from build123d import *

# Parameters (mm, degrees)
F0_W     = 127
F0_H     = 88.9
F1_DEPTH = 127
F2_R     = 5.08
F4_DEPTH = 114.3
F6_DEPTH = 10.16


with BuildPart() as f1:
    # F0 (on Top) → F1 (new body)
    with BuildSketch(Plane.XY):
        with Locations((4.240815, 7.625027)):
            Rectangle(F0_W, F0_H)
    extrude(amount=F1_DEPTH)

    # F2
    f2_edges = [f1.edges().sort_by_distance(p)[0] for p in [
        (-59.259185, -36.824973, 63.5),
        (67.740815, -36.824973, 63.5),
        (67.740815, 52.075027, 63.5),
        (-59.259185, 52.075027, 63.5),
    ]]
    fillet(f2_edges, radius=F2_R)

    # F3 (on face) → F4 (cut)
    with BuildSketch(Plane.XY.offset(127)):
        with BuildLine():
            Line((58.850815, 49.535027), (-50.369185, 49.535027))
            ThreePointArc((-50.369185, 49.535027), (-54.859313, 47.675155), (-56.719185, 43.185027))
            Line((-56.719185, 43.185027), (-56.719185, -27.934973))
            ThreePointArc((-56.719185, -27.934973), (-54.859313, -32.425101), (-50.369185, -34.284973))
            Line((-50.369185, -34.284973), (58.850815, -34.284973))
            ThreePointArc((58.850815, -34.284973), (63.340943, -32.425101), (65.200815, -27.934973))
            Line((65.200815, -27.934973), (65.200815, 43.185027))
            ThreePointArc((65.200815, 43.185027), (63.340943, 47.675155), (58.850815, 49.535027))
        make_face()
    extrude(amount=-F4_DEPTH, mode=Mode.SUBTRACT)

    # F5 (on face) → F6 (cut)
    with BuildSketch(Plane(origin=(0, 0, 0), x_dir=(1, 0, 0), z_dir=(0, 0, -1))):
        with BuildLine():
            ThreePointArc((58.850815, -49.535027), (63.340943, -47.675155), (65.200815, -43.185027))
            Line((65.200815, -43.185027), (65.200815, 27.934973))
            ThreePointArc((65.200815, 27.934973), (63.340943, 32.425101), (58.850815, 34.284973))
            Line((58.850815, 34.284973), (-50.369185, 34.284973))
            ThreePointArc((-50.369185, 34.284973), (-54.859313, 32.425101), (-56.719185, 27.934973))
            Line((-56.719185, 27.934973), (-56.719185, -43.185027))
            ThreePointArc((-56.719185, -43.185027), (-54.859313, -47.675155), (-50.369185, -49.535027))
            Line((-50.369185, -49.535027), (58.850815, -49.535027))
        make_face()
    extrude(amount=-F6_DEPTH, mode=Mode.SUBTRACT)


solid = f1.part
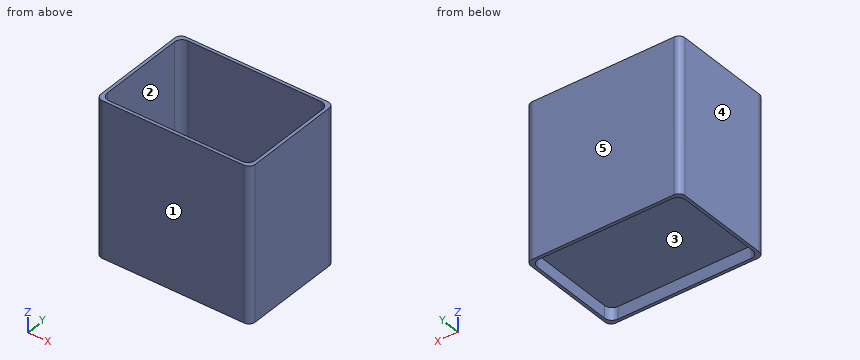
Here's how the part is built. I have some questions about the finished solid (model axes, mm). Face numbers are marked on the shaded views. A direction names the side the tool comes from. Round coordinates to 2 decimals unless told otherwise and drop trailing zeros. Order: outer loops, then holes, each group sorted by start corner. A loop starts at its lowest first (then second) coordinate and runs counter-clockwise, first axis right, second up. Notation, with made-up numbers: (-27.5, 66.5) -> (11.5, 66.5) arc R17 ccw to (11.5, 96.5) -> close; hole circle Ø9 at (4.25, 68.25). An arc over 180 degrees is marked (long way). Return JSON: item names as keys, results as strings.
Q1. If we mould it in two halves opening along Y, with no side actions, what happens to the marked faces 3, 4 and 5? For each: released by +Y, released by -Y, zero draft, split by the parting line, or undercut.
Filled sheet:
{"face 3": "undercut", "face 4": "zero draft", "face 5": "released by +Y"}
Q2. For pin 1 Ø8 at (x, y) = (-44.5, 22.5) entering from +Z; pin 2 Ø2 at (x, y) = (-17, 15) entering from -Z, each with a flat end and sliding along its axis, tell me the tip position at first contact or that it passes through.
Filled sheet:
{"pin 1": "stops at z = 12.7", "pin 2": "stops at z = 10.16"}
Q3. If we section it at A-A on z = 118.5: List the corners of the cut face in (x, y) for me, plus the area to 3 significant figures.
Filled sheet:
{"outline": "(-59.26, -31.74) arc R5.08 ccw to (-54.18, -36.82) -> (62.66, -36.82) arc R5.08 ccw to (67.74, -31.74) -> (67.74, 47) arc R5.08 ccw to (62.66, 52.08) -> (-54.18, 52.08) arc R5.08 ccw to (-59.26, 47) -> close; hole (-56.72, -27.93) arc R6.35 ccw to (-50.37, -34.28) -> (58.85, -34.28) arc R6.35 ccw to (65.2, -27.93) -> (65.2, 43.19) arc R6.35 ccw to (58.85, 49.54) -> (-50.37, 49.54) arc R6.35 ccw to (-56.72, 43.19) -> close", "area": "1,080 mm^2"}
Q4. Which directions (+Z, -Z, +X, -X, +Y, -Y) give clear straight access to the entire face, cutting with the end or side of a thin tool? Please do the marked faces 1 and 2.
Filled sheet:
{"face 1": "+Z, -Z, +X, -X, -Y", "face 2": "+Z"}
Q5. I need wall thicknesses on line 1 along X through (y, z) = (-24, 14); line 2 along Y through (x, z) = (27, 66); line 3 along Z through (x, y) = (11.5, 24). Which ranges of each line are inside material? Lowest first, please. Write a range as from..to.
Filled sheet:
{"line 1": "x = -59.26..-56.72, 65.2..67.74", "line 2": "y = -36.82..-34.28, 49.54..52.08", "line 3": "z = 10.16..12.7"}
Q6. If we section it at B-B on x = 48.5: List the corners of the cut face in (y, z) for me.
Filled sheet:
{"outline": "(-36.82, 0) -> (-34.28, 0) -> (-34.28, 10.16) -> (49.54, 10.16) -> (49.54, 0) -> (52.08, 0) -> (52.08, 127) -> (49.54, 127) -> (49.54, 12.7) -> (-34.28, 12.7) -> (-34.28, 127) -> (-36.82, 127) -> close"}
Q7. If we section it at C-C on y = -3: List the corners of the cut face in (x, z) for me.
Filled sheet:
{"outline": "(-59.26, 0) -> (-56.72, 0) -> (-56.72, 10.16) -> (65.2, 10.16) -> (65.2, 0) -> (67.74, 0) -> (67.74, 127) -> (65.2, 127) -> (65.2, 12.7) -> (-56.72, 12.7) -> (-56.72, 127) -> (-59.26, 127) -> close"}
